from build123d import *

# Parameters (mm, degrees)
BOSS_EXTRUDE1_DEPTH      = 2
BOSS_EXTRUDE1_DEPTH_BACK = 2
SKETCH1_R                = 1.75
SKETCH1_R_2              = 11.25
SKETCH2_W                = 42
SKETCH2_H                = 4
BOSS_EXTRUDE2_DEPTH      = 45
FILLET4_R                = 2
SKETCH3_R                = 1.75
CUT_EXTRUDE1_DEPTH       = 10
SKETCH3_4_R              = 1.75
CUT_EXTRUDE2_DEPTH       = 2.5
SKETCH10_R               = 3.05
BOSS_EXTRUDE4_DEPTH      = 4
SKETCH11_W               = 58
SKETCH11_H               = 4
BOSS_EXTRUDE5_DEPTH      = 24
SKETCH12_R               = 1.75
CUT_EXTRUDE3_DEPTH       = 24
SKETCH12_3_R             = 1.75
CUT_EXTRUDE4_DEPTH       = 2.5
FILLET5_R                = 2.5
BOSS_EXTRUDE6_DEPTH      = 2
LPATTERN1_COUNT          = 2
LPATTERN1_PITCH          = 51
FILLET6_R                = 2.5
FILLET7_R                = 2.5
FILLET7_OF_MIRROR3_R     = 2.5
SKETCH15_W               = 3.203134656
SKETCH15_H               = 5.191613013
BOSS_EXTRUDE7_DEPTH      = 4
FILLET8_R                = 2.5


with BuildPart() as part:
    # Sketch1 → Boss-Extrude1 (new, two sides: drawn at the far end of the back side and taken through both)
    with BuildSketch(Plane(origin=(0, 0, 0), x_dir=(0, 0, -1), z_dir=(1, 0, 0)).offset(-BOSS_EXTRUDE1_DEPTH_BACK)):
        with BuildLine():
            Line((-16, 21), (16, 21))
            ThreePointArc((16, 21), (19.535533906, 19.535533906), (21, 16))
            Line((21, 16), (21, -21))
            Line((21, -21), (-21, -21))
            Line((-21, -21), (-21, 16))
            ThreePointArc((-21, 16), (-19.535533906, 19.535533906), (-16, 21))
        make_face()
        with Locations((15.5, 15.5)):
            Circle(SKETCH1_R, mode=Mode.SUBTRACT)
        with Locations(Location((-15.5, 15.5, 0), (0, 0, 180))):
            Circle(SKETCH1_R, mode=Mode.SUBTRACT)
        with Locations(Location((15.5, -15.5, 0), (0, 0, 180))):
            Circle(SKETCH1_R, mode=Mode.SUBTRACT)
        with Locations((-15.5, -15.5)):
            Circle(SKETCH1_R, mode=Mode.SUBTRACT)
        Circle(SKETCH1_R_2, mode=Mode.SUBTRACT)
    extrude(amount=BOSS_EXTRUDE1_DEPTH + BOSS_EXTRUDE1_DEPTH_BACK)

    # Sketch2 → Boss-Extrude2 (add)
    with BuildSketch(Plane.ZY.offset(2)):
        with Locations((0, -23)):
            Rectangle(SKETCH2_W, SKETCH2_H)
    extrude(amount=-BOSS_EXTRUDE2_DEPTH)

    # Fillet4
    fillet4_edges = [part.edges().sort_by_distance(p)[0] for p in [
        (43, -23, -21),
        (43, -23, 21),
    ]]
    fillet(fillet4_edges, radius=FILLET4_R)

    # Sketch3 → Cut-Extrude1 (cut)
    with BuildSketch(Plane(origin=(0, -21, 0), x_dir=(1, 0, 0), z_dir=(0, 1, 0))):
        with Locations(Location((37.777001089, 15.480581557, 0), (0, 0, 270))):
            Circle(SKETCH3_R)
        with Locations(Location((37.777001089, -15.519418443, 0), (0, 0, 270))):
            Circle(SKETCH3_R)
        with Locations(Location((6.777001089, -15.519418443, 0), (0, 0, 270))):
            Circle(SKETCH3_R)
        with Locations(Location((6.777001089, 15.480581557, 0), (0, 0, 270))):
            Circle(SKETCH3_R)
    extrude(amount=-CUT_EXTRUDE1_DEPTH, mode=Mode.SUBTRACT)

    # Sketch3<4> → Cut-Extrude2 (cut)
    # profile 1 of 4: a face of its own
    with BuildSketch(Plane(origin=(0, -21, 0), x_dir=(1, 0, 0), z_dir=(0, 1, 0))):
        Polygon((37.777001089, -18.810314977), (40.627001089, -17.16486671), (40.627001089, -13.873970176), (37.777001089, -12.228521908), (34.927001089, -13.873970176), (34.927001089, -17.16486671), align=None)
        with Locations(Location((37.777001089, -15.519418443, 0), (0, 0, 270))):
            Circle(SKETCH3_4_R, mode=Mode.SUBTRACT)
    # profile 2 of 4: a face of its own
    with BuildSketch(Plane(origin=(0, -21, 0), x_dir=(1, 0, 0), z_dir=(0, 1, 0))):
        Polygon((5.131552822, -18.369418443), (8.422449356, -18.369418443), (10.067897623, -15.519418443), (8.422449356, -12.669418443), (5.131552822, -12.669418443), (3.486104555, -15.519418443), align=None)
        with Locations(Location((6.777001089, -15.519418443, 0), (0, 0, 270))):
            Circle(SKETCH3_4_R, mode=Mode.SUBTRACT)
    # profile 3 of 4: a face of its own
    with BuildSketch(Plane(origin=(0, -21, 0), x_dir=(1, 0, 0), z_dir=(0, 1, 0))):
        Polygon((40.627001089, 13.83513329), (40.627001089, 17.126029824), (37.777001089, 18.771478092), (34.927001089, 17.126029824), (34.927001089, 13.83513329), (37.777001089, 12.189685023), align=None)
        with Locations(Location((37.777001089, 15.480581557, 0), (0, 0, 270))):
            Circle(SKETCH3_4_R, mode=Mode.SUBTRACT)
    # profile 4 of 4: a face of its own
    with BuildSketch(Plane(origin=(0, -21, 0), x_dir=(1, 0, 0), z_dir=(0, 1, 0))):
        Polygon((5.131552822, 12.630581557), (8.422449356, 12.630581557), (10.067897623, 15.480581557), (8.422449356, 18.330581557), (5.131552822, 18.330581557), (3.486104555, 15.480581557), align=None)
        with Locations(Location((6.777001089, 15.480581557, 0), (0, 0, 270))):
            Circle(SKETCH3_4_R, mode=Mode.SUBTRACT)
    extrude(amount=-CUT_EXTRUDE2_DEPTH, mode=Mode.SUBTRACT)

    # Sketch10 → Boss-Extrude4 (add)
    with BuildSketch(Plane.ZY.offset(2)):
        with BuildLine():
            Line((16, 21), (21, 21))
            Line((21, 21), (74, 21))
            ThreePointArc((74, 21), (77.535533906, 19.535533906), (79, 16))
            Line((79, 16), (79, -25))
            Line((79, -25), (21, -25))
            Line((21, -25), (21, 16))
            Line((21, 16), (16, 21))
        make_face()
        with Locations((50, 0)):
            Circle(SKETCH10_R, mode=Mode.SUBTRACT)
    extrude(amount=-BOSS_EXTRUDE4_DEPTH)

    # Sketch11 → Boss-Extrude5 (add)
    with BuildSketch(Plane(origin=(2, 0, 0), x_dir=(0, 0, -1), z_dir=(1, 0, 0))):
        with Locations((-50, -23)):
            Rectangle(SKETCH11_W, SKETCH11_H)
    extrude(amount=BOSS_EXTRUDE5_DEPTH)

    # Sketch12 → Cut-Extrude3 (cut)
    with BuildSketch(Plane(origin=(0, -21, 0), x_dir=(1, 0, 0), z_dir=(0, 1, 0))):
        with Locations(Location((7.297001089, -38.019418443, 0), (0, 0, 270))):
            Circle(SKETCH12_R)
        with Locations(Location((7.297001089, -66.019418443, 0), (0, 0, 270))):
            Circle(SKETCH12_R)
    extrude(amount=-CUT_EXTRUDE3_DEPTH, mode=Mode.SUBTRACT)

    # Sketch12<3> → Cut-Extrude4 (cut)
    # profile 1 of 2: a face of its own
    with BuildSketch(Plane(origin=(0, -21, 0), x_dir=(1, 0, 0), z_dir=(0, 1, 0))):
        Polygon((5.651552822, -40.869418443), (8.942449356, -40.869418443), (10.587897623, -38.019418443), (8.942449356, -35.169418443), (5.651552822, -35.169418443), (4.006104555, -38.019418443), align=None)
        with Locations(Location((7.297001089, -38.019418443, 0), (0, 0, 270))):
            Circle(SKETCH12_3_R, mode=Mode.SUBTRACT)
    # profile 2 of 2: a face of its own
    with BuildSketch(Plane(origin=(0, -21, 0), x_dir=(1, 0, 0), z_dir=(0, 1, 0))):
        Polygon((5.651552822, -68.869418443), (8.942449356, -68.869418443), (10.587897623, -66.019418443), (8.942449356, -63.169418443), (5.651552822, -63.169418443), (4.006104555, -66.019418443), align=None)
        with Locations(Location((7.297001089, -66.019418443, 0), (0, 0, 270))):
            Circle(SKETCH12_3_R, mode=Mode.SUBTRACT)
    extrude(amount=-CUT_EXTRUDE4_DEPTH, mode=Mode.SUBTRACT)

    # Fillet5
    fillet5_edges = [part.edges().sort_by_distance(p)[0] for p in [
        (26, -23, 21),
        (26, -23, 79),
    ]]
    fillet(fillet5_edges, radius=FILLET5_R)

    # Sketch14 → Boss-Extrude6 (add)
    with BuildSketch(Plane(origin=(0, 0, -21), x_dir=(-1, 0, 0), z_dir=(0, 0, -1))):
        Polygon((-2, -2.5), (-21.5, -21), (-25.716216216, -21), (-25.716216216, -25), (2, -25), (2, 1.294871795), (-2, 1.294871795), align=None)
    boss_extrude6 = extrude(amount=BOSS_EXTRUDE6_DEPTH)

    # LPattern1: Boss-Extrude6 ×2
    with Locations(*[(0, 0, i * LPATTERN1_PITCH) for i in range(1, LPATTERN1_COUNT)]):
        add(boss_extrude6)

    # Fillet6
    # the kernel refuses this fillet: 2.5 mm, written as the material it takes off along each edge
    with BuildSketch(Plane(origin=(25.716216216, -14.876275643, -23), x_dir=(-1, 0, 0), z_dir=(0, -1, 0))) as fillet6_piece_1:
        with BuildLine():
            CenterArc((2.449489743, -2.5), FILLET6_R, 90, 78.463040967)
            Line((0, -2), (-0.048989795, -1.99))
            ThreePointArc((-0.048989795, -1.99), (-0.05, -1), (-0.05, 0))
            Line((-0.05, 0), (0, 0.05))
            Line((0, 0.05), (2.449489743, 0.05))
            Line((2.449489743, 0.05), (2.449489743, 0))
        make_face()
    extrude(amount=16.247448714, mode=Mode.SUBTRACT)

    # Fillet7
    # the kernel refuses this fillet: 2.5 mm, written as the material it takes off along each edge
    with BuildSketch(Plane(origin=(-8.123724357, 1.294871795, -23), x_dir=(0, -1, 0), z_dir=(1, 0, 0))) as fillet7_piece_1:
        with BuildLine():
            CenterArc((2.449489743, -2.5), FILLET7_R, 90, 78.463040967)
            Line((0, -2), (-0.048989795, -1.99))
            ThreePointArc((-0.048989795, -1.99), (-0.05, -1), (-0.05, 0))
            Line((-0.05, 0), (0, 0.05))
            Line((0, 0.05), (2.449489743, 0.05))
            Line((2.449489743, 0.05), (2.449489743, 0))
        make_face()
    extrude(amount=16.247448714, mode=Mode.SUBTRACT)

    # Mirror3: Boss-Extrude6 across plane
    add(boss_extrude6.mirror(Plane.XY.offset(29)))

    # Fillet7 of Mirror3
    # the kernel refuses this fillet: 2.5 mm, written as the material it takes off along each edge
    with BuildSketch(Plane(origin=(-8.123724357, 1.294871795, 81), x_dir=(0, -1.5735190928007313e-12, -1.0), z_dir=(1, 0, 0))) as fillet7_of_mirror3_piece_1:
        with BuildLine():
            CenterArc((2.5, -2.449489743), FILLET7_OF_MIRROR3_R, 101.536959033, 78.463040967)
            Line((0, -2.449489743), (-0.05, -2.449489743))
            Line((-0.05, -2.449489743), (-0.05, 0))
            Line((-0.05, 0), (0, 0.05))
            ThreePointArc((0, 0.05), (1, 0.05), (1.99, 0.048989795))
            Line((1.99, 0.048989795), (2, 0))
        make_face()
    extrude(amount=16.247448714, mode=Mode.SUBTRACT)

    # Sketch15 → Boss-Extrude7 (add)
    with BuildSketch(Plane(origin=(0, -21, 0), x_dir=(1, 0, 0), z_dir=(0, 1, 0))):
        with Locations((24.398432672, -78.404193494)):
            Rectangle(SKETCH15_W, SKETCH15_H)
    extrude(amount=-BOSS_EXTRUDE7_DEPTH)

    # Fillet8
    fillet8_edges = [part.edges().sort_by_distance(p)[0] for p in [
        (26, -23, 81),
    ]]
    fillet(fillet8_edges, radius=FILLET8_R)


solid = part.part
Verification items for the finished model (mm, model axes). A direction names the side the tool comes from. Coordinates: 2 decimals unless noted, no trailing zeros. Write each loop counter-clockwise with the first axis right and the second up, starting at its lowest first coordinate (ties: lowest second). Pieces come first, ordered by that corner, then holes. Notation, with made-up numbers: (59.5, 77) - (80.5, 77) arc R16 ccw to (80.5, 104) - close; hole circle Ø1 at (-11, 65). An arc over 180 degrees is marked (long way). Answer as a JSON object with one key per item and string values.
(1) Cross-section at C-C on y = -6. Record the cut outline in (x, z).
Report:
{"outline": "(-2, -23) - (5.69, -23) - (5.69, -21) - (2, -21) - (2, -9.52) - (-2, -9.52) - close; (-2, 9.52) - (2, 9.52) - (2, 28) - (5.69, 28) - (5.69, 30) - (2, 30) - (2, 79) - (5.69, 79) - (5.69, 81) - (-2, 81) - close"}
(2) Cross-section at A-A on z = 50. Record the cut outline in (x, y), plus the area to 3 significant figures.
Report:
{"outline": "(-2, -25) - (26, -25) - (26, -21) - (2, -21) - (2, -3.05) - (-2, -3.05) - close; (-2, 3.05) - (2, 3.05) - (2, 21) - (-2, 21) - close", "area": "256 mm^2"}
(3) Tool access check on faces 1 (the flat face through (33, -23, -21)), 2 (the cylindrical face through (39.51, -24.24, -15.71)), 3 (the flat face through (40.627, -22, 16)), 4 (the cylindrical face through (-0.03, -9.98, -5.19)), 5 (the flat face through (0, 9, -21)). Record the directions out of +Z, -Z, +X, -X, +Y, -Y that give a thin tool (end or side, any length) a straight path to the whole face; none if there is none.
Report:
{"face 1": "-Z, +X, +Y, -Y", "face 2": "+Y, -Y", "face 3": "+Y", "face 4": "+X, -X", "face 5": "-Z, +X, -X, +Y"}
(4) Cross-section at D-D on z = 25. Record the cut outline in (x, y).
Report:
{"outline": "(-2, -25) - (26, -25) - (26, -21) - (2, -21) - (2, 21) - (-2, 21) - close"}
(5) Cross-section at B-B on y = 0. Record the cut outline in (x, z), plus the area to 3 significant figures.
Report:
{"outline": "(-2, -22.72) - (2, -22.72) - (2, -11.25) - (-2, -11.25) - close; (-2, 11.25) - (2, 11.25) - (2, 46.95) - (-2, 46.95) - close; (-2, 53.05) - (2, 53.05) - (2, 80.72) - (-2, 80.72) - close", "area": "299 mm^2"}
(6) Gauge pin test, flat ends, axial feed: pin 1 Ø4 at (y, z) = (-1, 33.5) entering from +X; pin 2 Ø1.5 at (x, z) = (7, 40.5) entering from +Y; pin 3 Ø3 at (x, z) = (8, 15.5) entering from +Y. Record the tip position at first contact, or that the pin passes through.
Report:
{"pin 1": "x = 2", "pin 2": "y = -21", "pin 3": "y = -23.5"}
(7) Mould release check, pull along X, two halves, no side actions. Record for faces 6 (the cylindrical face through (26.713, -22.972, 21.752)), 7 (the cylindrical face through (6.627, -24.24, 39.636)), 8 (the flat face through (18, -21, 17)): pulls with the +X half, pulls with the -X half, needs draft (parallel to the pull), parting line crosses it, or undercut.
Report:
{"face 6": "pulls with the +X half", "face 7": "undercut", "face 8": "needs draft"}
(8) Thickness scan on line 1 along Y through (x, z) = (8, 44.5); line 2 along X through (y, z) = (-20.5, 11); line 3 along Z through (x, y) = (0, 15). Record the ranges inside material, lowest first.
Report:
{"line 1": "-25 to -21", "line 2": "-2 to 2", "line 3": "-21 to -17.18, -13.82 to 13.82, 17.18 to 79"}
